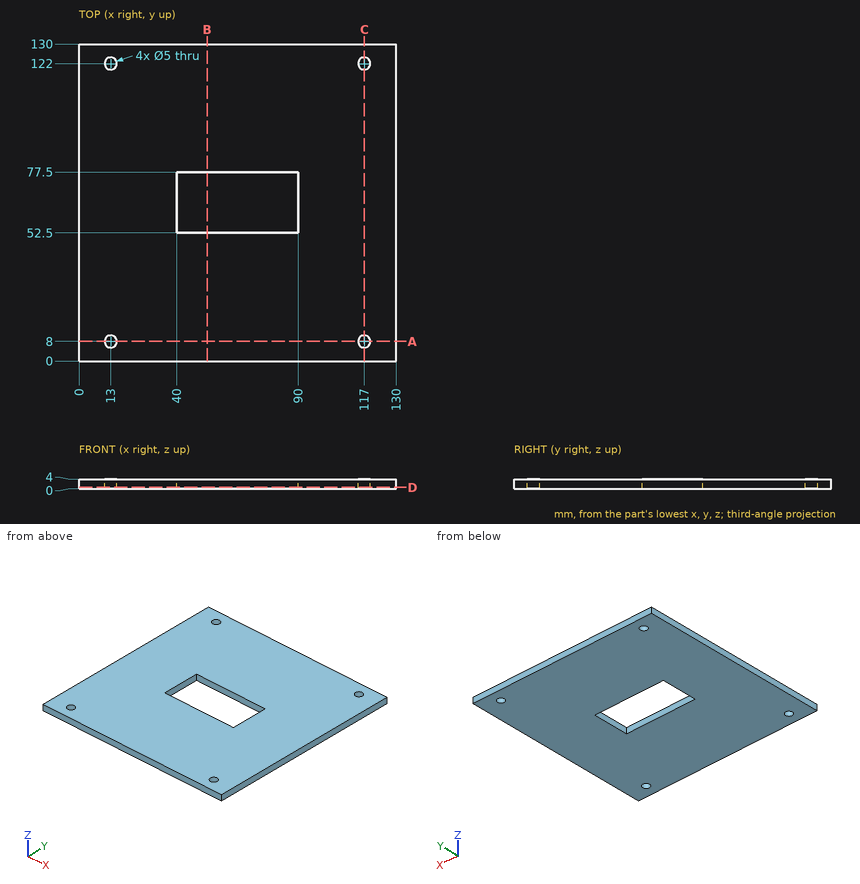
Here's the drawing with two shaded views (mm, measured from the low corner). I have some questions. Round coordinates to 2 decimals unless told otherwise and drop trailing zeros. Loops run counter-clockwise (first coordinate to the right, second up) from the corner with the lowest first, then second, coordinate; pieces in that order, holes last. Notation, with made-up numbers: M 80,49 L 114,49 A32 ccw 114,75 Z; hole C -8,26.25 d6. An arc over 180 degrees is marked long. Answer as a JSON object with one key per item and string values. Group by question number.
Q1. Imagine slicing it at B-B, the plane x = 52.5. Please give me the cut outline in (y, z).
Q2. Will this pin go through, and if not, where does the flat tip stop? pin 1 (3 mm diameter, centred on x = 117, y = 8, fed in from -Z).
Q3. Please list where these lines run through material, in increasing order: L1, parallel to Y at x = 13, z = 2.8; L2, parallel to X at y = 69, z = 3.7; L3, parallel to Y at x = 60, z = 2.05.
Q4. Imagine slicing it at D-D, the plane z = 0.6. Please give me the cut outline in (x, y).
Q5. Imagine slicing it at A-A, the plane y = 8. Please give me the cut outline in (x, z).
Q6. Imagine slicing it at C-C, the plane x = 117. Please give me the cut outline in (y, z).
Findings:
{
 "1": {"outline": "M 0,0 L 52.5,0 L 52.5,4 L 0,4 Z; M 77.5,0 L 130,0 L 130,4 L 77.5,4 Z"},
 "2": {"pin 1": "passes through"},
 "3": {"L1": "y = 0 to 5.5, 10.5 to 119.5, 124.5 to 130", "L2": "x = 0 to 40, 90 to 130", "L3": "y = 0 to 52.5, 77.5 to 130"},
 "4": {"outline": "M 0,0 L 130,0 L 130,130 L 0,130 Z; hole C 13,8 d5; hole C 13,122 d5; hole M 40,52.5 L 90,52.5 L 90,77.5 L 40,77.5 Z; hole C 117,8 d5; hole C 117,122 d5"},
 "5": {"outline": "M 0,0 L 10.5,0 L 10.5,4 L 0,4 Z; M 15.5,0 L 114.5,0 L 114.5,4 L 15.5,4 Z; M 119.5,0 L 130,0 L 130,4 L 119.5,4 Z"},
 "6": {"outline": "M 0,0 L 5.5,0 L 5.5,4 L 0,4 Z; M 10.5,0 L 119.5,0 L 119.5,4 L 10.5,4 Z; M 124.5,0 L 130,0 L 130,4 L 124.5,4 Z"}
}
